Print and shaded views of the part. All mm, measured from the part's lowest x, y and z. A direction names the side the tool comes from. Round coordinates to 2 decimals unless told otherwise and drop trailing zeros. Loops run counter-clockwise (first coordinate to the right, second up) from the corner with the lowest first, then second, coordinate; pieces in that order, holes last. Notation, with made-up numbers: (25.25, -11) - (47.25, -11) arc R17 ccw to (47.25, 12) - close; hole circle Ø11 at (84, 48). An arc over 180 degrees is marked (long way). Answer as a JSON object with one key per item and string values.
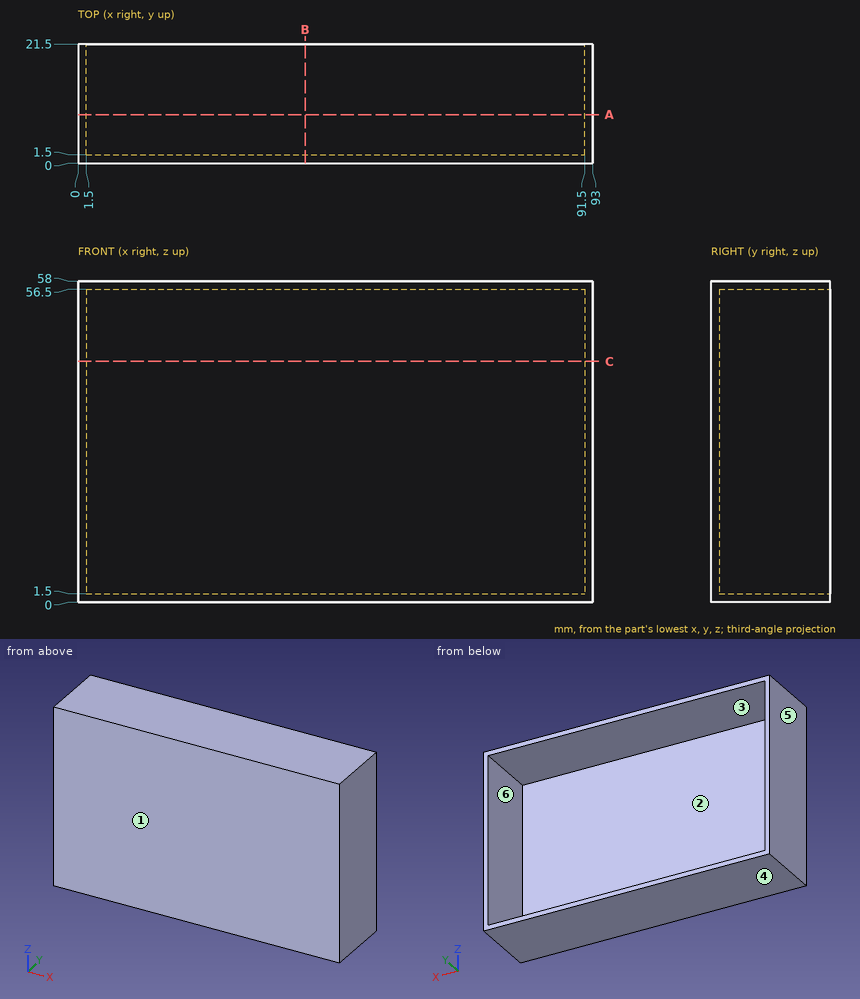
1) Drop flat-ended pins along their axis: P1, Ø6, axis at x = 32.5, z = 48, coming from the +Y side; P2, Ø3, axis at x = 61.5, y = 14, coming from the -Z side. Give the stop position or say it passes through.
Values follow:
{"P1": "y = 1.5", "P2": "z = 0"}
2) Slice it at A-A on y = 8.75. List the corners of the cut face in (x, z), then the cut area to 3 significant figures.
Values follow:
{"outline": "(0, 0) - (93, 0) - (93, 58) - (0, 58) - close; hole (1.5, 1.5) - (91.5, 1.5) - (91.5, 56.5) - (1.5, 56.5) - close", "area": "444 mm²"}
3) Slice it at B-B on x = 41. List the corners of the cut face in (y, z), then the cut area to 3 significant figures.
Values follow:
{"outline": "(0, 0) - (21.5, 0) - (21.5, 1.5) - (1.5, 1.5) - (1.5, 56.5) - (21.5, 56.5) - (21.5, 58) - (0, 58) - close", "area": "147 mm²"}
4) Two-plate mould, pull along X, no slides. Class the marked faces 3, 4, 5 and 6: pulls with the +X half, pulls with the -X half, needs draft (parallel to the pull), parting line crosses it, or undercut.
Values follow:
{"face 3": "undercut", "face 4": "needs draft", "face 5": "pulls with the -X half", "face 6": "undercut"}
5) Slice it at C-C on z = 43.5. List the corners of the cut face in (x, y), then the cut area to 4 significant figures.
Values follow:
{"outline": "(0, 0) - (93, 0) - (93, 21.5) - (91.5, 21.5) - (91.5, 1.5) - (1.5, 1.5) - (1.5, 21.5) - (0, 21.5) - close", "area": "199.5 mm²"}
6) Tool access for the marked faces 1 and 2: list every direction of +Z, -Z, +X, -X, +Y, -Y with a clear straight run to the whole face (end or side of a thin tool).
Values follow:
{"face 1": "+Z, -Z, +X, -X, -Y", "face 2": "+Y"}
7) Probe probe 1 along Z at (x, y) = (48.5, 9); probe 2 along X at (y, z) = (19.5, 15); probe 3 along Y at (x, z) = (64, 31). List the from-to ranges inside material, lowest first.
Values follow:
{"probe 1": "0 to 1.5, 56.5 to 58", "probe 2": "0 to 1.5, 91.5 to 93", "probe 3": "0 to 1.5"}
